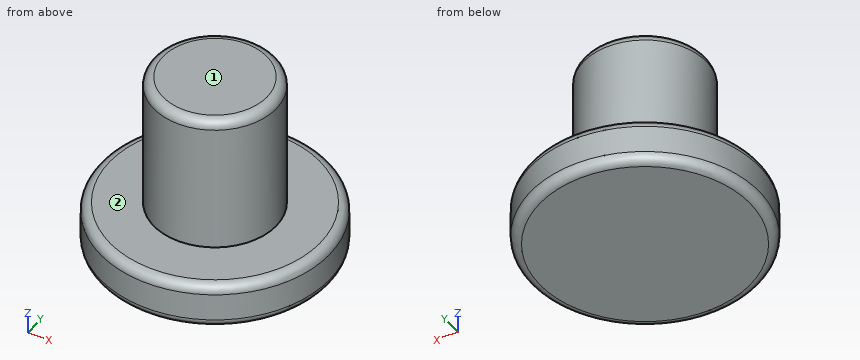
from build123d import *

# Parameters (mm, degrees)
F0_R     = 12.5
F1_DEPTH = 5
F2_R     = 6.7
F3_DEPTH = 20
F4_R     = 1


with BuildPart() as f1:
    # F0 (on Top) → F1 (new body)
    with BuildSketch(Plane.XY):
        Circle(F0_R)
    extrude(amount=F1_DEPTH)

    # F2 (on face) → F3 (join)
    with BuildSketch(Plane(origin=(0, 0, 0), x_dir=(1, 0, 0), z_dir=(0, 0, -1))):
        Circle(F2_R)
    extrude(amount=-F3_DEPTH)

    # F4
    f4_edges = [f1.edges().sort_by_distance(p)[0] for p in [
        (-12.5, 0, 0),
        (-12.5, 0, 5),
        (-6.7, 0, 20),
    ]]
    fillet(f4_edges, radius=F4_R)


solid = f1.part
Model file for the job. Use its own axes, mm. Face numbers are marked on the shaded views. A direction names the side the tool comes from. Give positions to 0.01 mm unless a question says otherwise; leave off trailing zeros. Write each loop counter-clockwise with the first axis right and the second up, starting at its lowest first coordinate (ties: lowest second). Pieces come first, ordered by that corner, then holes. Notation, with made-up numbers: (51, -33) - (55, -33) arc R14 ccw to (55, -20) - close; hole circle Ø6 at (51.5, 34.25). An arc over 180 degrees is marked (long way). Answer as CSV lines item,"result".
1. Drill centre lines: L1, parallel to Y at x = 0, z = 6.5; L2, parallel to Z at x = 3.75, y = 5.75; L3, parallel to Y at x = -5.75, z = 6.25. Where is each one in solid material? Low to high. Write a range as [from, to].
Responses:
L1,"y = [-6.7, 6.7]"
L2,"z = [0, 5]"
L3,"y = [-3.44, 3.44]"
2. Band-saw the part on A-A (y = 0). Write the cut outline in (x, z), and give its area (3 significant figures).
Responses:
outline,"(-12.5, 1) arc R1 ccw to (-11.5, 0) - (11.5, 0) arc R1 ccw to (12.5, 1) - (12.5, 4) arc R1 ccw to (11.5, 5) - (6.7, 5) - (6.7, 19) arc R1 ccw to (5.7, 20) - (-5.7, 20) arc R1 ccw to (-6.7, 19) - (-6.7, 5) - (-11.5, 5) arc R1 ccw to (-12.5, 4) - close"
area,"325 mm2"
3. Band-saw the part on C-C (z = 2.5). Write the cut outline in (x, y), and give its area (3 significant figures).
Responses:
outline,"circle Ø25 at (0, 0)"
area,"491 mm2"
4. Pin check, flat tips, straight feed: pin 1 (8 mm diameter, centred on x = -1.5, y = 9, fed in from -Z); pin 2 (3 mm diameter, centred on x = -6, z = 14.5, fed in from +Y); pin 3 (8 mm diameter, centred on y = -1.5, z = 14.5, fed in from +X); pin 4 (4 mm diameter, centred on y = 8, z = 2, fed in from +X). Stop position of each tip, or through.
Responses:
pin 1,"stops at z = 0"
pin 2,"stops at y = 4.96"
pin 3,"stops at x = 6.7"
pin 4,"stops at x = 10.97"
5. Band-saw the part on D-D (z = 5.75). Write the cut outline in (x, y), and give its area (3 significant figures).
Responses:
outline,"circle Ø13.4 at (0, 0)"
area,"141 mm2"
6. 3-axis set-ups, long thin cutter, end or side, ignore diameter. For the marked faces 1 and 2: which of +Z, -Z, +X, -X, +Y, -Y reach the whole face in a straight line?
Responses:
face 1,"+Z, +X, -X, +Y, -Y"
face 2,"+Z"
